Could you check a few things on this model? Use its own coordinates, in mm. Give positions to 0.01 mm unless a question says otherwise; leave off trailing zeros. Write each loop counter-clockwise with the first axis right and the second up, starting at its lowest first coordinate (ties: lowest second). Pieces come first, ordered by that corner, then holes. Notation, with made-up numbers: M 67,26 L 95,26 A34 ccw 95,63 Z; hole C 70,22 d3. An arc over 180 degrees is marked long. One line per item, written item: value.
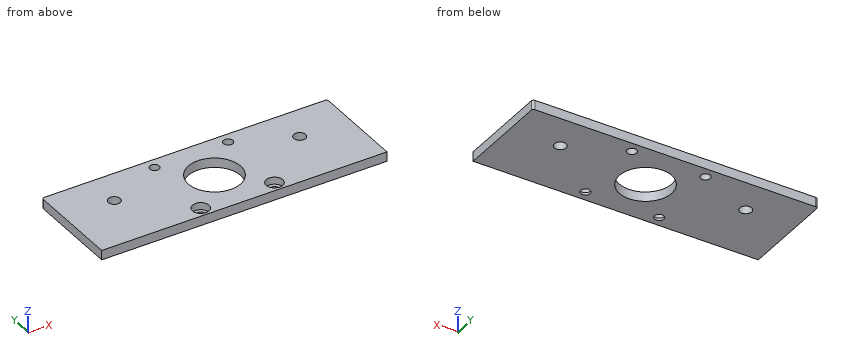
```python
from build123d import *

# Parameters (mm, degrees)
SKETCH1_W           = 120
SKETCH1_H           = 40
SKETCH1_R           = 2.5
SKETCH1_R_2         = 11
SKETCH1_R_3         = 2
BOSS_EXTRUDE1_DEPTH = 4
FILLET1_R           = 1
SKETCH2_R           = 3.5
CUT_EXTRUDE1_DEPTH  = 3


with BuildPart() as part:
    # Sketch1 → Boss-Extrude1 (new body)
    with BuildSketch(Plane.XY):
        with Locations((60, 20)):
            Rectangle(SKETCH1_W, SKETCH1_H)
        with Locations((21, 25)):
            Circle(SKETCH1_R, mode=Mode.SUBTRACT)
        with Locations((99, 25)):
            Circle(SKETCH1_R, mode=Mode.SUBTRACT)
        with Locations((60, 20)):
            Circle(SKETCH1_R_2, mode=Mode.SUBTRACT)
        with Locations((75.5, 35.5)):
            Circle(SKETCH1_R_3, mode=Mode.SUBTRACT)
        with Locations((75.5, 4.5)):
            Circle(SKETCH1_R_3, mode=Mode.SUBTRACT)
        with Locations((44.5, 4.5)):
            Circle(SKETCH1_R_3, mode=Mode.SUBTRACT)
        with Locations((44.5, 35.5)):
            Circle(SKETCH1_R_3, mode=Mode.SUBTRACT)
    extrude(amount=BOSS_EXTRUDE1_DEPTH)

    # Fillet1
    fillet1_edges = [part.edges().sort_by_distance(p)[0] for p in [
        (0, 40, 2),
        (120, 40, 2),
    ]]
    fillet(fillet1_edges, radius=FILLET1_R)

    # Sketch2 → Cut-Extrude1 (cut)
    with BuildSketch(Plane.XY.offset(4)):
        with Locations((44.5, 4.5)):
            Circle(SKETCH2_R)
        with Locations((75.5, 4.5)):
            Circle(SKETCH2_R)
    extrude(amount=-CUT_EXTRUDE1_DEPTH, mode=Mode.SUBTRACT)


solid = part.part
```
1) Please list where these lines run through material, in increasing order: L1, parallel to Y at x = 75.5, z = 2; L2, parallel to X at y = 26.5, z = 3.65; L3, parallel to Y at x = 21, z = 1.6. Write a range as from..to.
Outcome:
L1: y = 0..1, 8..33.5, 37.5..40
L2: x = 0..19, 23..51.13, 68.87..97, 101..120
L3: y = 0..22.5, 27.5..40
2) If we section it at D-D, the plane x = 21: Write out the boundary of the cut face in (y, z), then the cut area to 3 significant figures.
Outcome:
outline: M 0,0 L 22.5,0 L 22.5,4 L 0,4 Z; M 27.5,0 L 40,0 L 40,4 L 27.5,4 Z
area: 140 mm^2
3) I'm going to push flat-ended pins straight in: pin 1 (8 mm diameter, centred on x = 99, y = 25, fed in from +Z); pin 2 (2 mm diameter, centred on x = 76.5, y = 5, fed in from +Z). Where does each tip first touch, or does it pass through?
Outcome:
pin 1: stops at z = 4
pin 2: stops at z = 1
4) If we section it at C-C, the plane z = 2.5: Write out the boundary of the cut face in (x, y), then the cut area to 3 significant figures.
Outcome:
outline: M 0,0 L 120,0 L 120,39 A1 ccw 119,40 L 1,40 A1 ccw 0,39 Z; hole C 21,25 d5; hole C 44.5,4.5 d7; hole C 44.5,35.5 d4; hole C 60,20 d22; hole C 75.5,4.5 d7; hole C 75.5,35.5 d4; hole C 99,25 d5
area: 4,280 mm^2
5) If we section it at A-A, the plane y = 4.5: Write out the boundary of the cut face in (x, z), then the cut area to 3 significant figures.
Outcome:
outline: M 0,0 L 42.5,0 L 42.5,1 L 41,1 L 41,4 L 0,4 Z; M 46.5,0 L 73.5,0 L 73.5,1 L 72,1 L 72,4 L 48,4 L 48,1 L 46.5,1 Z; M 77.5,0 L 120,0 L 120,4 L 79,4 L 79,1 L 77.5,1 Z
area: 430 mm^2
6) If we section it at B-B, the plane x = 44.5: Write out the boundary of the cut face in (y, z).
Outcome:
outline: M 0,0 L 2.5,0 L 2.5,1 L 1,1 L 1,4 L 0,4 Z; M 6.5,0 L 33.5,0 L 33.5,4 L 8,4 L 8,1 L 6.5,1 Z; M 37.5,0 L 40,0 L 40,4 L 37.5,4 Z
